For this review, take the finished solid that the model builds, in its own axes (mm). Face numbers are marked on the shaded views. A direction names the side the tool comes from. Give positions to 0.01 mm unless a question says otherwise; leave off trailing zeros.
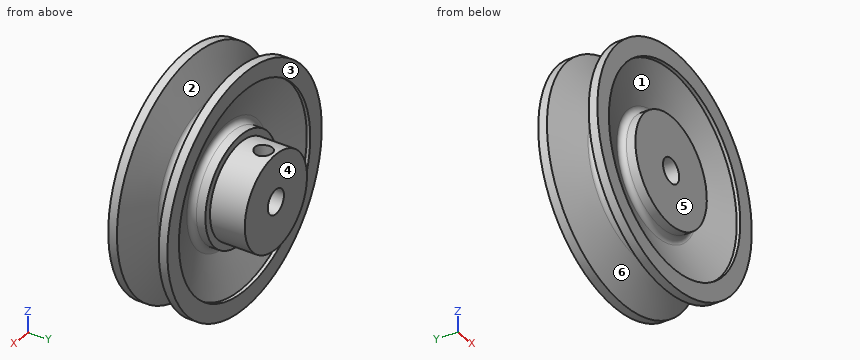
```python
from build123d import *

# Parameters (mm, degrees)
CUT_EXTRUDE1_START = 4.898979378
CUT_EXTRUDE1_DEPTH = 22.101020701


# Read off the part's stored shape, not the designer's step: Cut-Extrude1
with BuildPart() as part:
    # Sketch1 → Revolve1 (revolve)
    with BuildSketch(Plane.XY, mode=Mode.PRIVATE) as revolve1_sk:
        with BuildLine():
            Line((-7, 50), (-27, 50))
            Line((-27, 50), (-27, 30))
            Line((-27, 30), (-31, 30))
            Line((-31, 30), (-31, 24.821217929))
            ThreePointArc((-31, 24.821217929), (-32.279270691, 22.363761796), (-35.02606043, 22.002140067))
            Line((-35.02606043, 22.002140067), (-57, 30))
            Line((-57, 30), (-57, 32))
            Line((-57, 32), (-67, 32))
            Line((-67, 32), (-67, 27))
            Line((-67, 27), (-43.97393957, 18.619199391))
            ThreePointArc((-43.97393957, 18.619199391), (-42.542543867, 17.520850838), (-42, 15.800121529))
            Line((-42, 15.800121529), (-42, 14.199878471))
            ThreePointArc((-42, 14.199878471), (-42.542543867, 12.479149162), (-43.97393957, 11.380800609))
            Line((-43.97393957, 11.380800609), (-67, 3))
            Line((-67, 3), (-67, -2))
            Line((-67, -2), (-57, -2))
            Line((-57, -2), (-57, 0))
            Line((-57, 0), (-35.02606043, 7.997859933))
            ThreePointArc((-35.02606043, 7.997859933), (-32.279270691, 7.636238204), (-31, 5.178782071))
            Line((-31, 5.178782071), (-31, 0))
            Line((-31, 0), (-7, 0))
            Line((-7, 0), (-7, 50))
        make_face()
    revolve(revolve1_sk.sketch.rotate(Axis((0, 0, 0), (0, 1, 0)), 270), axis=Axis((0, 0, 0), (0, 1, 0)))

    # Cut-Extrude1 outline → Cut-Extrude1 (cut)
    with BuildSketch(Plane.XY.offset(CUT_EXTRUDE1_START)):
        with BuildLine():
            add(Edge.make_bspline(
                [(-5, 43), (-5, 41.67563617), (-4.455498311, 40.384216944), (-2.614748823, 38.543894661), (-1.310387974, 38.000764057), (1.304550701, 37.999237646), (2.604262767, 38.533632867), (4.465141201, 40.393635869), (4.999476778, 41.691327392), (5.000522421, 44.30467144), (4.459732186, 45.609641922), (2.617817368, 47.4549382), (1.324771948, 47.999010031), (-1.31728863, 48.000987169), (-2.612604689, 47.457113982), (-4.45328192, 45.61913124), (-5, 44.32436383), (-5, 43)],
                knots=[0, 0, 0, 0, 0.125, 0.125, 0.25, 0.25, 0.375, 0.375, 0.5, 0.5, 0.625, 0.625, 0.75, 0.75, 0.875, 0.875, 1, 1, 1, 1], degree=3))
        make_face()
    extrude(amount=CUT_EXTRUDE1_DEPTH, mode=Mode.SUBTRACT)


solid = part.part
```
Q1. For pin 1 Ø18.5 at (x, z) = (4, 1) entering from -Y; pin 2 Ø3 at (x, z) = (42, -17) entering from -Y; pin 3 Ø6 at (y, z) = (37.5, 10.5) entering from +X, all flat-tipped, find the tip position at first contact; note any pin that passes through.
Answers:
pin 1: stops at y = 0
pin 2: stops at y = 3.71
pin 3: stops at x = 25.94
Q2. Mouldability with a two-part tool opening along X and no side actions: class the marked faces 4, 5 and 6 as +X half, -X half, draft (parallel to the pull), parting line (faces both ways), or undercut.
Answers:
face 4: draft
face 5: undercut
face 6: parting line
Q3. Consider section A-A on x = 0. Count the separate pieces of the cut face and the enclosed holes in it, plus the area to 3 significant figures.
Answers:
separate pieces: 3
enclosed holes: 0
area: 3,060 mm2
Q4. For probe 1 along X at (y, z) = (31.5, 0); probe 2 along X at (y, z) = (-1, 0); probe 3 along X at (y, z) = (15, 0), list the stretches that pass through material, from the lowest coordinate up.
Answers:
probe 1: x = -67 to -57, -27 to -7, 7 to 27, 57 to 67
probe 2: x = -67 to -57, 57 to 67
probe 3: x = -42 to -7, 7 to 42
Q5. Machinability: for the marked faces 1, 2 and 3, which of the approach directions +Z, -Z, +X, -X, +Y, -Y give a long, thin tool a straight path to every point of the face, cutting with its end or side? Answer none if there is none.
Answers:
face 1: -Y
face 2: none
face 3: +Y
